```python
from build123d import *

# Parameters (mm, degrees)
SKETCH1_R           = 2
BOSS_EXTRUDE1_DEPTH = 1.524
FILLET1_R           = 1


with BuildPart() as part:
    # Sketch1 → Boss-Extrude1 (new body, symmetric)
    with BuildSketch(Plane(origin=(0, 0, 0), x_dir=(1, 0, 0), z_dir=(0, 1, 0))):
        with BuildLine():
            Line((-26.418872232, 3.81), (26.418872232, 3.81))
            ThreePointArc((26.418872232, 3.81), (30.228872232, 0), (26.418872232, -3.81))
            Line((26.418872232, -3.81), (-26.418872232, -3.81))
            ThreePointArc((-26.418872232, -3.81), (-30.228872232, 0), (-26.418872232, 3.81))
        make_face()
        with Locations((-26.418872232, 0)):
            Circle(SKETCH1_R, mode=Mode.SUBTRACT)
        with Locations((26.418872232, 0)):
            Circle(SKETCH1_R, mode=Mode.SUBTRACT)
    extrude(amount=BOSS_EXTRUDE1_DEPTH, both=True)

    # Fillet1
    fillet1_edges = [part.edges().sort_by_distance(p)[0] for p in [
        (30.228872232, 1.524, 0),
        (0, 1.524, -3.81),
        (-30.228872232, 1.524, 0),
        (0, -1.524, -3.81),
        (30.228872232, -1.524, 0),
        (0, -1.524, 3.81),
        (-30.228872232, -1.524, 0),
        (0, 1.524, 3.81),
    ]]
    fillet(fillet1_edges, radius=FILLET1_R)


solid = part.part
```
For this review, take the finished solid that the model builds, in its own axes (mm). Round coordinates to 2 decimals unless told otherwise and drop trailing zeros. Write each loop counter-clockwise with the first axis right and the second up, starting at its lowest first coordinate (ties: lowest second). Pieces come first, ordered by that corner, then holes. Notation, with made-up numbers: (57, 7.5) - (90, 7.5) arc R25 ccw to (90, 37.5) - close; hole circle Ø11 at (84.5, 17). An arc over 180 degrees is marked (long way). Answer as a JSON object with one key per item and string values.
1. Draft analysis for pull direction X (two halves, no side actions). For faces 1 (the face through (28.327, -0.021, -0.601)), 2 (the face through (-30.23, 0.01, 0.08)), 3 (the face through (-0.37, -1.223, 3.525)), state which applies: +X half, -X half, draft (parallel to the pull), parting line (faces both ways), or undercut.
Response values:
{"face 1": "undercut", "face 2": "-X half", "face 3": "draft"}
2. To check wall thickness, follow line 1 along X through (y, z) = (0.4, 0); line 2 along X through (y, z) = (0, -1.5); line 3 along Z through (x, y) = (-25.5, -1.2). State the ranges of each line that lie inside material, in increasing order.
Response values:
{"line 1": "x = -30.23 to -28.42, -24.42 to 24.42, 28.42 to 30.23", "line 2": "x = -29.92 to -27.74, -25.1 to 25.1, 27.74 to 29.92", "line 3": "z = -3.55 to -1.78, 1.78 to 3.55"}
3. We need section C-C on y = 1.05. Give the boundary of the cut face in (x, z).
Response values:
{"outline": "(-26.42, -3.66) - (26.42, -3.66) arc R3.66 ccw to (26.42, 3.66) - (-26.42, 3.66) arc R3.66 ccw to start; hole circle Ø4 at (-26.42, 0); hole circle Ø4 at (26.42, 0)"}
4. We need section A-A on z = 0. Give the boundary of the cut face in (x, y).
Response values:
{"outline": "(-30.23, -0.52) arc R1 ccw to (-29.23, -1.52) - (-28.42, -1.52) - (-28.42, 1.52) - (-29.23, 1.52) arc R1 ccw to (-30.23, 0.52) - close; (-24.42, -1.52) - (24.42, -1.52) - (24.42, 1.52) - (-24.42, 1.52) - close; (28.42, -1.52) - (29.23, -1.52) arc R1 ccw to (30.23, -0.52) - (30.23, 0.52) arc R1 ccw to (29.23, 1.52) - (28.42, 1.52) - close"}
5. We need section B-B on x = -6. Give the boundary of the cut face in (y, z).
Response values:
{"outline": "(-1.52, -2.81) arc R1 ccw to (-0.52, -3.81) - (0.52, -3.81) arc R1 ccw to (1.52, -2.81) - (1.52, 2.81) arc R1 ccw to (0.52, 3.81) - (-0.52, 3.81) arc R1 ccw to (-1.52, 2.81) - close"}
